from build123d import *

# Parameters (mm, degrees)
F1_DEPTH = 101.6
F4_DEPTH = 127
F6_DEPTH = 76.2


with BuildPart() as f1:
    # F0 (on Top) → F1 (new body)
    with BuildSketch(Plane.XY):
        Polygon((-63.5, 14.05588), (-38.1, -62.14412), (38.1, -62.14412), (63.5, 14.05588), align=None)
    extrude(amount=F1_DEPTH)

    # F3 (on offset) → F4 (cut)
    with BuildSketch(Plane.YZ.offset(63.5)):
        with BuildLine():
            Line((-2.288038, 110.407464), (-33.979441, 110.407464))
            ThreePointArc((-33.979441, 110.407464), (-46.417855, 109.443983), (-57.741659, 104.208156))
            Line((-57.741659, 104.208156), (-68.357266, 104.208156))
            Line((-68.357266, 104.208156), (-68.357266, 91.704749))
            Line((-68.357266, 91.704749), (-68.357266, 52.956361))
            Line((-68.357266, 52.956361), (-62.043723, 52.956361))
            ThreePointArc((-62.043723, 52.956361), (-27.599395, 50.705769), (-2.288038, 74.175155))
            Line((-2.288038, 74.175155), (-2.288038, 110.407464))
        make_face()
    extrude(amount=-F4_DEPTH, mode=Mode.SUBTRACT)

    # F5 (on Top) → F6 (cut)
    with BuildSketch(Plane.XY):
        Polygon((55.033333, 7.70588), (-55.033333, 7.70588), (-33.866667, -55.79412), (33.866667, -55.79412), align=None)
    extrude(amount=F6_DEPTH, mode=Mode.SUBTRACT)


solid = f1.part
Part model, mm, in its own coordinate system. A direction names the side the tool comes from. Coordinates: 2 decimals unless noted, no trailing zeros. Order: outer loops, then holes, each group sorted by start corner. A loop starts at its lowest first (then second) coordinate and runs counter-clockwise, first axis right, second up.
(1) Slice it at A-A, the plane z = 10. Write the cut outline in (x, y).
Check sheet entries:
outline: (-63.5, 14.06) - (-38.1, -62.14) - (38.1, -62.14) - (63.5, 14.06) - close; hole (-55.03, 7.71) - (-33.87, -55.79) - (33.87, -55.79) - (55.03, 7.71) - close
(2) Pin check, flat tips, straight feed: pin 1 Ø6 at (y, z) = (-10, 17.5) entering from -X; pin 2 Ø3 at (x, y) = (26.5, 4) entering from -Z; pin 3 Ø22 at (x, z) = (5.5, 82) entering from -Y. Stop position of each tip, or through.
Check sheet entries:
pin 1: stops at x = -56.48
pin 2: stops at z = 76.2
pin 3: stops at y = -2.29
(3) Tool access for faces 4 (the face through (0, -55.794, 25)), 5 (the face through (1, -2.288, 88)), 6 (the face through (1, 7.706, 38)), 7 (the face through (0, 10, 0)): list every direction of +Z, -Z, +X, -X, +Y, -Y with a clear straight run to the whole face (end or side of a thin tool).
Check sheet entries:
face 4: +Z, -Z
face 5: +Z, +X, -X, -Y
face 6: -Z
face 7: -Z, +X, -X, +Y, -Y
(4) Slice it at B-B, the plane x = -23.5. Write the cut outline in (y, z).
Check sheet entries:
outline: (-62.14, 0) - (-55.79, 0) - (-55.79, 50.36) arc R43.65 cw to (-62.04, 52.96) - (-62.14, 52.96) - close; (-2.29, 76.2) - (7.71, 76.2) - (7.71, 0) - (14.06, 0) - (14.06, 101.6) - (-2.29, 101.6) - close
(5) Slice it at D-D, the plane y = -50. Write the cut outline in (x, z).
Check sheet entries:
outline: (-42.15, 0) - (-35.8, 0) - (-35.8, 48.89) - (-42.15, 48.89) - close; (35.8, 0) - (42.15, 0) - (42.15, 48.89) - (35.8, 48.89) - close
(6) Pull direction X, two halves, no side cores. Call faces 1 (the face through (53.444, -16.111, 38.8)), 2 (the face through (-1, -62.144, 26)), 3 (the face through (44.3, -24.5, 29.1)): pulls with the +X half, pulls with the -X half, needs draft (parallel to the pull), parting line crosses it, or undercut.
Check sheet entries:
face 1: pulls with the +X half
face 2: needs draft
face 3: undercut
(7) Slice it at C-C, the plane y = -36. Write the cut outline in (x, z), and give its area (3 significant figures).
Check sheet entries:
outline: (-46.81, 0) - (-40.46, 0) - (-40.46, 48.63) - (-46.81, 48.63) - close; (40.46, 0) - (46.81, 0) - (46.81, 48.63) - (40.46, 48.63) - close
area: 618 mm2
(8) Probe L1, parallel to Y at x = 4.5, z = 50; L2, parallel to X at y = -33.5, z = 42; L3, parallel to Y at x = -49.5, z = 96. List the from-to ranges inside material, lowest first.
Check sheet entries:
L1: y = -62.14 to -55.79, 7.71 to 14.06
L2: x = -47.65 to -41.3, 41.3 to 47.65
L3: y = -2.29 to 14.06
